```python
from build123d import *

# Parameters (mm, degrees)
SKETCH1_R           = 3.35
SKETCH1_R_2         = 3.4
BOSS_EXTRUDE1_DEPTH = 20
SKETCH2_W           = 231.929502284
SKETCH2_H           = 220.245456765
BOSS_EXTRUDE2_DEPTH = 20
SKETCH3_W           = 20
SKETCH3_H           = 220.245456765
BOSS_EXTRUDE3_DEPTH = 150
SKETCH4_W           = 20
SKETCH4_H           = 220.245456765
BOSS_EXTRUDE4_DEPTH = 100
SKETCH5_R           = 20
BOSS_EXTRUDE5_DEPTH = 500


with BuildPart() as part:
    # Sketch1 → Boss-Extrude1 (new body)
    with BuildSketch(Plane.ZY.offset(22937.011755361)):
        Polygon((41237.494779256, 5557.929358856), (40773.575398624, 5106.753906388), (40825.939297891, 5052.910933366), (41289.858678523, 5504.086385835), align=None)
        with Locations((41221.902000531, 5502.053605549)):
            Circle(SKETCH1_R, mode=Mode.SUBTRACT)
        with Locations((41236.044136152, 5516.195741176)):
            Circle(SKETCH1_R, mode=Mode.SUBTRACT)
        with Locations((40870.597048417, 5108.322246569)):
            Circle(SKETCH1_R_2, mode=Mode.SUBTRACT)
        with Locations((40828.170641545, 5065.895839698)):
            Circle(SKETCH1_R_2, mode=Mode.SUBTRACT)
        with Locations((40828.170641545, 5150.74865344)):
            Circle(SKETCH1_R_2, mode=Mode.SUBTRACT)
        with Locations((40785.744234674, 5108.322246569)):
            Circle(SKETCH1_R_2, mode=Mode.SUBTRACT)
    extrude(amount=BOSS_EXTRUDE1_DEPTH)

    # Sketch2 → Boss-Extrude2 (add)
    with BuildSketch(Plane.ZY.offset(22957.011755361)):
        with Locations((40904.599781001, 5268.565849628)):
            Rectangle(SKETCH2_W, SKETCH2_H)
    extrude(amount=BOSS_EXTRUDE2_DEPTH)

    # Sketch3 → Boss-Extrude3 (add)
    with BuildSketch(Plane.ZY.offset(22957.011755361)):
        with Locations((40778.635029859, 5268.565849628)):
            Rectangle(SKETCH3_W, SKETCH3_H)
    extrude(amount=BOSS_EXTRUDE3_DEPTH)

    # Sketch4 → Boss-Extrude4 (add)
    with BuildSketch(Plane.XY.offset(40788.635029859)):
        with Locations((-23097.01175536, 5268.565849628)):
            Rectangle(SKETCH4_W, SKETCH4_H)
    extrude(amount=BOSS_EXTRUDE4_DEPTH)

    # Sketch5 → Boss-Extrude5 (add)
    with BuildSketch(Plane.XY.offset(40788.635029859)):
        with Locations((-23032.01175536, 5268.565849628)):
            Circle(SKETCH5_R)
    extrude(amount=BOSS_EXTRUDE5_DEPTH)


solid = part.part
```
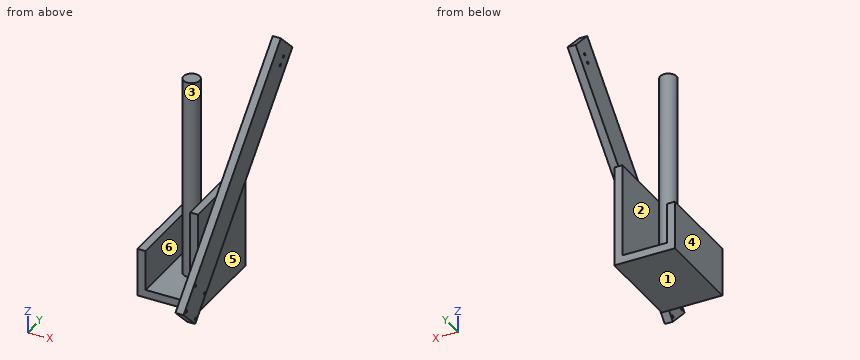
Check sheet for the modelled part. Datum: model origin and axes. Units: mm. Face numbers are marked on the shaded views. A direction names the side the tool comes from. Round coordinates to 2 decimals unless told otherwise and drop trailing zeros. Loops run counter-clockwise (first coordinate to the right, second up) from the corner with the lowest first, then second, coordinate; pieces in that order, holes last. Notation, with made-up numbers: (34, 42.25) -> (47, 42.25) arc R17 cw to (47, 53.25) -> close; hole circle Ø4 at (67.5, 57.25). An arc over 180 degrees is marked (long way). Answer in a Markdown table with one row per item.
Q1. Go/stop test with flat-tipped pins: P1, Ø10, axis at x = -23058, z = 41190, coming from the -Y side; P2, Ø20, axis at x = -23024, y = 5263, coming from the +Z side (3 decimals); P3, Ø11, axis at y = 5108.32, z = 40785.74, coming from the +X side; P4, Ø22, axis at x = -23095, y = 5236, coming from the +Z side (3 decimals). Record where each tip stops, or that it passes through.
Data:
| item | result |
|---|---|
| P1 | passes through |
| P2 | stops at z = 41288.635 |
| P3 | stops at x = -22937.01 |
| P4 | stops at z = 40888.635 |
Q2. Sectioned sample at A-A on z = 40845.5. Enter the section's corners in (x, y), then the cut area to 3 significant figures.
Data:
| item | result |
|---|---|
| outline | (-23107.01, 5158.44) -> (-23087.01, 5158.44) -> (-23087.01, 5378.69) -> (-23107.01, 5378.69) -> close; circle Ø40 at (-23032.01, 5268.57); (-22977.01, 5158.44) -> (-22957.01, 5158.44) -> (-22957.01, 5071.93) -> (-22937.01, 5071.93) -> (-22937.01, 5176.7) -> (-22957.01, 5176.7) -> (-22957.01, 5378.69) -> (-22977.01, 5378.69) -> close |
| area | 12,200 mm^2 |
Q3. Thickness scan on L1, parallel to X at y = 5348, z = 40793.5; L2, parallel to Z at x = -23025, y = 5333; L3, parallel to Z at x = -23091, y = 5233. Record the ranges inside material, lowest first.
Data:
| item | result |
|---|---|
| L1 | x = -23107.01 to -23087.01, -22977.01 to -22957.01 |
| L2 | z = 40768.64 to 40788.64 |
| L3 | z = 40768.64 to 40888.64 |
Q4. Set-up check for the marked faces 1, 2 and 3: record each of +Z, -Z, +X, -X, +Y, -Y from which the full face is reachable in a straight line by a thin tool's end or side.
Data:
| item | result |
|---|---|
| face 1 | -Z, +X, -X, +Y, -Y |
| face 2 | +Z, +Y, -Y |
| face 3 | +Z |
Q5. Sectioned sample at D-D on x = -23033. Enter the section's corners in (y, z), then the cut area to 3 significant figures.
Data:
| item | result |
|---|---|
| outline | (5158.44, 40768.64) -> (5378.69, 40768.64) -> (5378.69, 40788.64) -> (5288.54, 40788.64) -> (5288.54, 41288.64) -> (5248.59, 41288.64) -> (5248.59, 40788.64) -> (5158.44, 40788.64) -> close |
| area | 24,400 mm^2 |
Q6. Sectioned sample at C-C on z = 41078. Enter the section's corners in (x, y).
Data:
| item | result |
|---|---|
| outline | circle Ø40 at (-23032.01, 5268.57); (-22957.01, 5298.05) -> (-22937.01, 5298.05) -> (-22937.01, 5402.82) -> (-22957.01, 5402.82) -> close |
Q7. Sectioned sample at B-B on x = -22951. Enter the section's corners in (y, z).
Data:
| item | result |
|---|---|
| outline | (5052.91, 40825.94) -> (5106.75, 40773.58) -> (5557.93, 41237.49) -> (5504.09, 41289.86) -> close; hole circle Ø6.8 at (5065.9, 40828.17); hole circle Ø6.8 at (5108.32, 40785.74); hole circle Ø6.8 at (5108.32, 40870.6); hole circle Ø6.8 at (5150.75, 40828.17); hole circle Ø6.7 at (5502.05, 41221.9); hole circle Ø6.7 at (5516.2, 41236.04) |
Q8. Release check for a two-part mould opening along X. For the marked faces 4, 5 and 6 record: released by +X, released by -X, zero draft, split by the parting line, or undercut.
Data:
| item | result |
|---|---|
| face 4 | released by -X |
| face 5 | released by +X |
| face 6 | undercut |
